```python
from build123d import *

# Parameters (mm, degrees)
SKETCH1_W               = 154
SKETCH1_H               = 164
BOSS_EXTRUDE1_DEPTH     = 39
FILLET2_R               = 1
SKETCH2_R               = 5
SKETCH2_R_2             = 1
CUT_EXTRUDE1_DEPTH      = 37
CUT_EXTRUDE2_DEPTH      = 178.004271116
CUT_EXTRUDE2_DEPTH_BACK = 12.5
SKETCH3_R               = 5
SKETCH4_W               = 76
SKETCH4_H               = 41
CUT_EXTRUDE3_DEPTH      = 20
SKETCH5_W               = 80
SKETCH5_H               = 2
BOSS_EXTRUDE2_DEPTH     = 18
SKETCH7_W               = 85
SKETCH7_H               = 45
BOSS_EXTRUDE3_DEPTH     = 2
SKETCH8_W               = 18
SKETCH8_H               = 13
CUT_EXTRUDE4_DEPTH      = 3
SKETCH10_W              = 4
SKETCH10_H              = 51.783631986
BOSS_EXTRUDE4_DEPTH     = 20
SKETCH11_W              = 84.004327952
SKETCH11_H              = 44
CUT_EXTRUDE8_DEPTH      = 2
SKETCH12_W              = 4.408390859
SKETCH12_H              = 33
CUT_EXTRUDE9_DEPTH      = 3
SKETCH13_R              = 5
CUT_EXTRUDE10_DEPTH     = 10
SKETCH14_W              = 10
SKETCH14_H              = 5
CUT_EXTRUDE11_DEPTH     = 10
SKETCH15_R              = 1
CUT_EXTRUDE12_DEPTH     = 10


with BuildPart() as part:
    # Sketch1 → Boss-Extrude1 (new body)
    with BuildSketch(Plane(origin=(0, 0, 0), x_dir=(1, 0, 0), z_dir=(0, 1, 0))):
        with Locations((-25.679775281, -56.803370787)):
            Rectangle(SKETCH1_W, SKETCH1_H)
    extrude(amount=BOSS_EXTRUDE1_DEPTH)

    # Fillet2
    fillet2_edges = [part.edges().sort_by_distance(p)[0] for p in [
        (-25.679775281, 0, -25.196629213),
        (51.320224719, 0, 56.803370787),
        (-25.679775281, 0, 138.803370787),
        (-102.679775281, 0, 56.803370787),
    ]]
    fillet(fillet2_edges, radius=FILLET2_R)

    # Sketch2 → Cut-Extrude1 (cut)
    # profile 1 of 3: a face of its own
    with BuildSketch(Plane(origin=(0, 39, 0), x_dir=(1, 0, 0), z_dir=(0, 1, 0))):
        with BuildLine():
            Line((44.132250696, 23.196629213), (-96.23424538, 23.196629213))
            ThreePointArc((-96.23424538, 23.196629213), (-97.536310942, 20.053164875), (-100.679775281, 18.751099313))
            Line((-100.679775281, 18.751099313), (-100.679775281, -92.88384898))
            ThreePointArc((-100.679775281, -92.88384898), (-95.035253474, -98.528370787), (-100.679775281, -104.172892593))
            Line((-100.679775281, -104.172892593), (-100.679775281, -121.803370787))
            ThreePointArc((-100.679775281, -121.803370787), (-95.679775281, -126.803370787), (-100.679775281, -131.803370787))
            ThreePointArc((-100.679775281, -131.803370787), (-97.144241375, -133.267836881), (-95.679775281, -136.803370787))
            Line((-95.679775281, -136.803370787), (44.320224719, -136.803370787))
            ThreePointArc((44.320224719, -136.803370787), (45.784690813, -133.267836881), (49.320224719, -131.803370787))
            Line((49.320224719, -131.803370787), (49.320224719, 18.00865519))
            ThreePointArc((49.320224719, 18.00865519), (45.651773106, 19.528177601), (44.132250696, 23.196629213))
        make_face()
        with Locations(Location((-89.679775281, -2.276961684, 0), (0, 0, 270))):
            Circle(SKETCH2_R, mode=Mode.SUBTRACT)
        with Locations(Location((38.320224719, -2.276961684, 0), (0, 0, 270))):
            Circle(SKETCH2_R, mode=Mode.SUBTRACT)
    # profile 2 of 3: a face of its own
    with BuildSketch(Plane(origin=(0, 39, 0), x_dir=(1, 0, 0), z_dir=(0, 1, 0))):
        with Locations(Location((-89.679775281, -2.276961684, 0), (0, 0, 270))):
            Circle(SKETCH2_R_2)
    # profile 3 of 3: a face of its own
    with BuildSketch(Plane(origin=(0, 39, 0), x_dir=(1, 0, 0), z_dir=(0, 1, 0))):
        with Locations(Location((38.320224719, -2.276961684, 0), (0, 0, 270))):
            Circle(SKETCH2_R_2)
    extrude(amount=-CUT_EXTRUDE1_DEPTH, mode=Mode.SUBTRACT)

    # Sketch3 → Cut-Extrude2 (cut, two sides: drawn at the far end of the back side and taken through both)
    with BuildSketch(Plane(origin=(0, 39, 0), x_dir=(1, 0, 0), z_dir=(0, 1, 0)).offset(-CUT_EXTRUDE2_DEPTH_BACK)):
        with Locations(Location((-89.679775281, -2.276961684, 0), (0, 0, 270))):
            Circle(SKETCH3_R)
        with Locations(Location((38.320224719, -2.276961684, 0), (0, 0, 270))):
            Circle(SKETCH3_R)
        with BuildLine():
            Line((-100.679775281, -92.528370787), (-100.679775281, -104.528370787))
            ThreePointArc((-100.679775281, -104.528370787), (-94.679775281, -98.528370787), (-100.679775281, -92.528370787))
        make_face()
        with BuildLine():
            Line((-100.679775281, -121.803370787), (-100.679775281, -131.803370787))
            ThreePointArc((-100.679775281, -131.803370787), (-95.679775281, -126.803370787), (-100.679775281, -121.803370787))
        make_face()
    extrude(amount=CUT_EXTRUDE2_DEPTH + CUT_EXTRUDE2_DEPTH_BACK, mode=Mode.SUBTRACT)

    # Sketch4 → Cut-Extrude3 (cut)
    with BuildSketch(Plane.XZ):
        with Locations((9.320224719, 116.303370787)):
            Rectangle(SKETCH4_W, SKETCH4_H)
    extrude(amount=-CUT_EXTRUDE3_DEPTH, mode=Mode.SUBTRACT)

    # Sketch5 → Boss-Extrude2 (add)
    with BuildSketch(Plane(origin=(0, 2, 0), x_dir=(1, 0, 0), z_dir=(0, 1, 0))):
        with Locations((11.320224719, -94.803370787)):
            Rectangle(SKETCH5_W, SKETCH5_H)
        Polygon((-28.679775281, -95.803370787), (-28.679775281, -93.803370787), (-33.679775281, -93.803370787), (-33.679775281, -136.803370787), (-28.679775281, -136.803370787), align=None)
    extrude(amount=BOSS_EXTRUDE2_DEPTH)

    # Sketch7 → Boss-Extrude3 (add)
    with BuildSketch(Plane(origin=(0, 20, 0), x_dir=(1, 0, 0), z_dir=(0, 1, 0))):
        with Locations((8.820224719, -116.303370787)):
            Rectangle(SKETCH7_W, SKETCH7_H)
    extrude(amount=BOSS_EXTRUDE3_DEPTH)

    # Sketch8 → Cut-Extrude4 (cut)
    with BuildSketch(Plane(origin=(51.320224719, 0, 0), x_dir=(0, 0, -1), z_dir=(1, 0, 0))):
        with Locations((-117.065973314, 30.5)):
            Rectangle(SKETCH8_W, SKETCH8_H)
    extrude(amount=-CUT_EXTRUDE4_DEPTH, mode=Mode.SUBTRACT)

    # Sketch10 → Boss-Extrude4 (add)
    with BuildSketch(Plane.XZ):
        with Locations((49.320224719, 112.911554794)):
            Rectangle(SKETCH10_W, SKETCH10_H)
    extrude(amount=-BOSS_EXTRUDE4_DEPTH)

    # Sketch11 → Cut-Extrude8 (cut)
    with BuildSketch(Plane.XZ):
        with Locations((9.318060743, 116.803370787)):
            Rectangle(SKETCH11_W, SKETCH11_H)
    extrude(amount=-CUT_EXTRUDE8_DEPTH, mode=Mode.SUBTRACT)

    # Sketch12 → Cut-Extrude9 (cut)
    with BuildSketch(Plane(origin=(51.320224719, 0, 0), x_dir=(0, 0, -1), z_dir=(1, 0, 0))):
        with Locations((-52.479756675, 20.5)):
            Rectangle(SKETCH12_W, SKETCH12_H)
        with Locations((-45.479756675, 20.5)):
            Rectangle(SKETCH12_W, SKETCH12_H)
        with Locations((-38.479756675, 20.5)):
            Rectangle(SKETCH12_W, SKETCH12_H)
        with Locations((-31.479756676, 20.5)):
            Rectangle(SKETCH12_W, SKETCH12_H)
        with Locations((-24.479756676, 20.5)):
            Rectangle(SKETCH12_W, SKETCH12_H)
        with Locations((-17.479756675, 20.5)):
            Rectangle(SKETCH12_W, SKETCH12_H)
        with Locations((-10.479756676, 20.5)):
            Rectangle(SKETCH12_W, SKETCH12_H)
        with Locations((-3.479756676, 20.5)):
            Rectangle(SKETCH12_W, SKETCH12_H)
        with Locations((3.520243324, 20.5)):
            Rectangle(SKETCH12_W, SKETCH12_H)
        with Locations((10.520243325, 20.5)):
            Rectangle(SKETCH12_W, SKETCH12_H)
    extrude(amount=-CUT_EXTRUDE9_DEPTH, mode=Mode.SUBTRACT)

    # Sketch13 → Cut-Extrude10 (cut)
    with BuildSketch(Plane(origin=(0, 0, -25.196629213), x_dir=(-1, 0, 0), z_dir=(0, 0, -1))):
        with Locations((79.41479284, 31.5)):
            Circle(SKETCH13_R)
    extrude(amount=-CUT_EXTRUDE10_DEPTH, mode=Mode.SUBTRACT)

    # Sketch14 → Cut-Extrude11 (cut)
    with BuildSketch(Plane.ZY.offset(102.679775281)):
        with Locations((104.532679505, 31.835930774)):
            Rectangle(SKETCH14_W, SKETCH14_H)
    extrude(amount=-CUT_EXTRUDE11_DEPTH, mode=Mode.SUBTRACT)

    # Sketch15 → Cut-Extrude12 (cut)
    with BuildSketch(Plane.XZ.offset(-2)):
        with Locations(Location((-30.684103233, 116.803370787, 0), (0, 0, 270))):
            Circle(SKETCH15_R)
        with Locations(Location((49.320224719, 116.803370787, 0), (0, 0, 270))):
            Circle(SKETCH15_R)
    extrude(amount=-CUT_EXTRUDE12_DEPTH, mode=Mode.SUBTRACT)


solid = part.part
```
Geometry check sheet. Reference: the model listing, model coordinates, mm. A direction names the side the tool comes from. Give positions to 0.01 mm unless a question says otherwise; leave off trailing zeros. Write each loop counter-clockwise with the first axis right and the second up, starting at its lowest first coordinate (ties: lowest second). Pieces come first, ordered by that corner, then holes.
1) Section check A-A, the plane x = -70. Record the boundary of the cut face in (y, z), and give its area (3 significant figures).
2) Section check B-B, the plane z = 80. Record the boundary of the cut face in (x, y).
3) Release check for a two-part mould opening along X. For faces 1 (the flat face through (51.32, 19, 56)), 2 (the flat face through (-26, 0, 56)), 3 (the flat face through (7, 22, 115)) record: pulls with the +X half, pulls with the -X half, needs draft (parallel to the pull), parting line crosses it, or undercut.
4) Material ranges on L1, parallel to Z at x = 22, y = 12; L2, parallel to X at y = 31.5, z = 89; L3, parallel to Z at x = -56.5, y = 35, recorded low to high.
5) Access from +Z, -Z, +X, -X, +Y, -Y to the whole of each face (thin tool, end or side, straight path). Record for faces 4 (the flat face through (47.32, 11, 90)), 5 (the flat face through (9, 20, 117)).
6) Section check C-C, the plane y = 31.5. State how many separate pieces and enclosed holes the cut face has, and give its area (3 significant figures).
7) Gauge pin test, flat ends, axial feed: pin 1 (4 mm diameter, centred on x = 3, z = 106.5, fed in from -Y); pin 2 (12 mm diameter, centred on x = -54.5, z = 76, fed in from +Y); pin 3 (1.6 mm diameter, centred on x = 50.5, z = 16.5, fed in from -Y); pin 4 (1 mm diameter, centred on y = 29.5, z = 52, fed in from +X). Record the tip position at first contact, or that the pin passes through.
Computed:
1. outline: (0, -24.2) arc R1 ccw to (1, -25.2) - (39, -25.2) - (39, -23.2) - (2, -23.2) - (2, 136.8) - (39, 136.8) - (39, 138.8) - (1, 138.8) arc R1 ccw to (0, 137.8) - close
1. area: 476 mm2
2. outline: (-102.68, 1) arc R1 ccw to (-101.68, 0) - (50.32, 0) arc R1 ccw to (51.32, 1) - (51.32, 39) - (49.32, 39) - (49.32, 2) - (-100.68, 2) - (-100.68, 39) - (-102.68, 39) - close
3. face 1: pulls with the +X half
3. face 2: needs draft
3. face 3: undercut
4. L1: z = -25.2 to -23.2, 93.8 to 95.8, 136.8 to 138.8
4. L2: x = -102.68 to -100.68, 49.32 to 51.32
4. L3: z = -25.2 to -23.2, 136.8 to 138.8
5. face 4: +Y
5. face 5: -Y
6. separate pieces: 13
6. enclosed holes: 0
6. area: 1,170 mm2
7. pin 1: stops at y = 20
7. pin 2: stops at y = 2
7. pin 3: stops at y = 0
7. pin 4: stops at x = -100.68
